For this review, take the finished solid that the model builds, in its own axes (mm). Round coordinates to 2 decimals unless told otherwise and drop trailing zeros. Write each loop counter-clockwise with the first axis right and the second up, starting at its lowest first coordinate (ties: lowest second). Pieces come first, ordered by that corner, then holes. Notation, with made-up numbers: (1.25, -1.75) - (28.25, -1.75) arc R11 cw to (28.25, 2.25) - close; hole circle Ø2 at (26, -32). An arc over 180 degrees is marked (long way). Answer in a Markdown table with one row per item. Add a question column.
from build123d import *

# Parameters (mm, degrees)
SALIENTE_EXTRUIR1_DEPTH = 3.5


with BuildPart() as part:
    # Croquis1 → Saliente-Extruir1 (new body)
    with BuildSketch(Plane.XY):
        with BuildLine():
            Line((-16.907663566, -60.708333333), (13.092336434, -60.708333333))
            Line((13.092336434, -60.708333333), (23.808162125, -26.40922872))
            ThreePointArc((23.808162125, -26.40922872), (25.135875005, -23.695116141), (25.592336434, -20.708333333))
            Line((25.592336434, -20.708333333), (25.592336434, 14.291666667))
            ThreePointArc((25.592336434, 14.291666667), (22.663404246, 21.362734479), (15.592336434, 24.291666667))
            Line((15.592336434, 24.291666667), (-19.407663566, 24.291666667))
            ThreePointArc((-19.407663566, 24.291666667), (-26.478731378, 21.362734479), (-29.407663566, 14.291666667))
            Line((-29.407663566, 14.291666667), (-29.407663566, -20.708333333))
            ThreePointArc((-29.407663566, -20.708333333), (-28.951202137, -23.695116141), (-27.623489258, -26.40922872))
            Line((-27.623489258, -26.40922872), (-16.907663566, -60.708333333))
        make_face()
    extrude(amount=SALIENTE_EXTRUIR1_DEPTH)


solid = part.part
Q1. Add section A-A on z = 2.45. State the section outline as (x, y) points.
Q2. To check wall thickness, follow probe 1 along X at (y, z) = (-23, 3.1); probe 2 along X at (y, z) = (-46, 1.25). State the ranges of each line that lie inside material, in increasing order.
Q3. Add section C-C on x = 18.5. State the section outline as (y, z) points.
Q4. Add section B-B on y = 17.5. State the section outline as (x, z) points.
Answer sheet:
| question | item | result |
|---|---|---|
| 1 | outline | (-29.41, -20.71) arc R10 ccw to (-27.62, -26.41) - (-16.91, -60.71) - (13.09, -60.71) - (23.81, -26.41) arc R10 ccw to (25.59, -20.71) - (25.59, 14.29) arc R10 ccw to (15.59, 24.29) - (-19.41, 24.29) arc R10 ccw to (-29.41, 14.29) - close |
| 2 | probe 1 | x = -29.14 to 25.33 |
| 2 | probe 2 | x = -21.5 to 17.69 |
| 3 | outline | (-43.4, 0) - (23.86, 0) - (23.86, 3.5) - (-43.4, 3.5) - close |
| 4 | outline | (-28.88, 0) - (25.06, 0) - (25.06, 3.5) - (-28.88, 3.5) - close |
